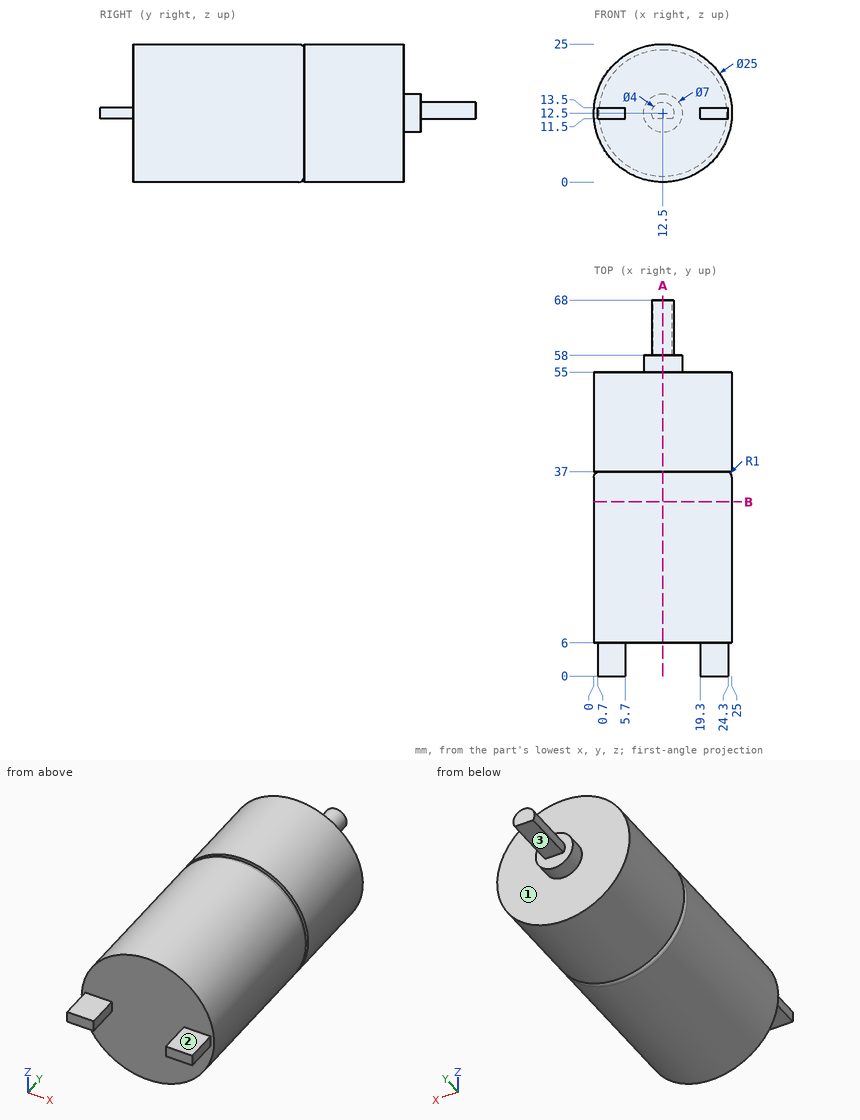
Check sheet for the drawn part. Datum: minimum x, y, z corner. Units: mm. A direction names the side the tool comes from. Coordinates: 2 decimals unless noted, no trailing zeros. Loops run counter-clockwise (first coordinate to the right, second up) from the corner with the lowest first, then second, coordinate; pieces in that order, holes last. Notation, with made-up numbers: (-1.75, 84.25) -> (31.25, 84.25) arc R23 ccw to (31.25, 106.25) -> close; hole circle Ø6 at (54.25, -1.75). An arc over 180 degrees is marked (long way). Answer as CSV lines item,"result".
1) Depth check by flat-ended pin: pin 1 (12 mm diameter, centred on x = 7.5, z = 6, fed in from +Y); pin 2 (4 mm diameter, centred on x = 21, y = 4.5, fed in from +Z); pin 3 (3 mm diameter, centred on y = 33, z = 22, fed in from +X). Enter the tip coordinate at first touch or a pass-through.
Found:
pin 1,"stops at y = 58"
pin 2,"stops at z = 22.73"
pin 3,"stops at x = 22.1"
2) Cross-section at A-A, the plane x = 12.5. Record the cut outline in (y, z).
Found:
outline,"(6, 0) -> (36, 0) arc R1 ccw to (37, 1) -> (37, 0) -> (55, 0) -> (55, 9) -> (58, 9) -> (58, 11.5) -> (68, 11.5) -> (68, 14.5) -> (58, 14.5) -> (58, 16) -> (55, 16) -> (55, 25) -> (37, 25) -> (37, 24) arc R1 ccw to (36, 25) -> (6, 25) -> close"
3) Cross-section at B-B, the plane y = 31.5. Record the cut outline in (x, z).
Found:
outline,"circle Ø25 at (12.5, 12.5)"
4) Tool access check on the marked faces 1, 2 and 3. Record the directions out of +Z, -Z, +X, -X, +Y, -Y that give a thin tool (end or side, any length) a straight path to the whole face; none if there is none.
Found:
face 1,"+Y"
face 2,"+Z, +X, -X, -Y"
face 3,"-Z, +X, -X, +Y"
5) Thickness scan on L1, parallel to Y at x = 14, z = 16.25; L2, parallel to Y at x = 12.5, z = 9.5; L3, parallel to Z at x = 21.25, y = 4.5. Record the ranges inside material, lowest first. Write a range as from..to.
Found:
L1,"y = 6..55"
L2,"y = 6..58"
L3,"z = 11.5..13.5"
